Work out the finished part from the listing and answer in its coordinate system (mm). A direction names the side the tool comes from. Round coordinates to 2 decimals unless told otherwise and drop trailing zeros. Write each loop counter-clockwise with the first axis right and the second up, starting at its lowest first coordinate (ties: lowest second). Pieces come first, ordered by that corner, then holes. Notation, with made-up numbers: M 75.5,24.25 L 96.5,24.25 A26 ccw 96.5,39.25 Z; hole C 42.25,6 d4. An arc over 180 degrees is marked long. Answer in a Markdown table with one row per item.
```python
from build123d import *

# Parameters (mm, degrees)
BOSS_EXTRUDE1_DEPTH     = 15
SKETCH2_R               = 10
CUT_EXTRUDE1_DEPTH      = 109.972473589
SKETCH3_W               = 40
SKETCH3_H               = 10
BOSS_EXTRUDE2_DEPTH     = 55
CUT_EXTRUDE2_DEPTH      = 136.738719605
CUT_EXTRUDE2_DEPTH_BACK = 136.738719605


with BuildPart() as part:
    # Sketch1 → Boss-Extrude1 (new body)
    with BuildSketch(Plane(origin=(0, 0, 0), x_dir=(1, 0, 0), z_dir=(0, 1, 0))):
        with BuildLine():
            Line((0, 25), (80, 25))
            ThreePointArc((80, 25), (105, 0), (80, -25))
            Line((80, -25), (0, -25))
            ThreePointArc((0, -25), (-25, 0), (0, 25))
        make_face()
    extrude(amount=BOSS_EXTRUDE1_DEPTH)

    # Sketch2 → Cut-Extrude1 (cut, through all)
    with BuildSketch(Plane(origin=(0, 15, 0), x_dir=(1, 0, 0), z_dir=(0, 1, 0))):
        with Locations(Location((0, 0, 0), (0, 0, 270))):
            Circle(SKETCH2_R)
        with Locations(Location((80, 0, 0), (0, 0, 90))):
            Circle(SKETCH2_R)
    extrude(amount=-CUT_EXTRUDE1_DEPTH, mode=Mode.SUBTRACT)

    # Sketch3 → Boss-Extrude2 (add)
    with BuildSketch(Plane(origin=(0, 15, 0), x_dir=(1, 0, 0), z_dir=(0, 1, 0))):
        with Locations((40, 20)):
            Rectangle(SKETCH3_W, SKETCH3_H)
        with Locations((40, -20)):
            Rectangle(SKETCH3_W, SKETCH3_H)
    extrude(amount=BOSS_EXTRUDE2_DEPTH)

    # Sketch4 → Cut-Extrude2 (cut, two sides)
    with BuildSketch(Plane.XY.offset(25)) as cut_extrude2_sk:
        with BuildLine():
            ThreePointArc((30, 50), (40, 40), (50, 50))
            Line((50, 50), (30, 50))
        make_face()
        with BuildLine():
            Line((30, 50), (50, 50))
            ThreePointArc((50, 50), (40, 60), (30, 50))
        make_face()
        with BuildLine():
            ThreePointArc((40, 70), (54.142135624, 64.142135624), (60, 50))
            Line((60, 50), (60, 70))
            Line((60, 70), (40, 70))
        make_face()
        with BuildLine():
            ThreePointArc((20, 50), (25.857864376, 64.142135624), (40, 70))
            Line((40, 70), (20, 70))
            Line((20, 70), (20, 50))
        make_face()
    extrude(amount=CUT_EXTRUDE2_DEPTH, mode=Mode.SUBTRACT)
    extrude(cut_extrude2_sk.sketch, amount=-CUT_EXTRUDE2_DEPTH_BACK, mode=Mode.SUBTRACT)


solid = part.part
```
1. A tool of negligible diameter and unlimited length cuts with its end or side. For faces 1 (the flat face through (40, 36, -15)), 2 (the flat face through (39, 27, -25)), 3 (the flat face through (20, 32, -20)), 4 (the cylindrical face through (37.83, 40.24, 20.07)), 5 (the flat face through (60, 32, 20)), from which of +Z, -Z, +X, -X, +Y, -Y can it reach the whole face along a straight path? Write none if from no direction.
Calculated:
| item | result |
|---|---|
| face 1 | +X, -X, +Y |
| face 2 | -Z, +X, -X, +Y, -Y |
| face 3 | +Z, -Z, -X, +Y |
| face 4 | +Z, -Z |
| face 5 | +Z, -Z, +X, +Y |
2. The part is cut by section C-C (y = 9). Determine the outline of the cut face in (x, z).
Calculated:
| item | result |
|---|---|
| outline | M 0,-25 L 80,-25 A25 ccw 80,25 L 0,25 A25 ccw Z; hole C 0,0 d20; hole C 80,0 d20 |
3. Determine the mould class of faces 6 (the flat face through (40, 36, 15)), 7 (the cylindrical face through (70.085, 7.605, 1.302)), 8 (the flat face through (20, 32, 20)) for opening direction X: released by +X, released by -X, zero draft, split by the parting line, or undercut.
Calculated:
| item | result |
|---|---|
| face 6 | zero draft |
| face 7 | undercut |
| face 8 | released by -X |
4. Consider line 1 along X through (y, z) = (9.5, 0); line 2 along Y through (x, z) = (40, 22.75); line 3 along X through (y, z) = (13.5, -8.5). Determine where each line is inside the solid, lowest interval first. Write a range as from..to.
Calculated:
| item | result |
|---|---|
| line 1 | x = -25..-10, 10..70, 90..105 |
| line 2 | y = 0..40, 60..70 |
| line 3 | x = -23.51..-5.27, 5.27..74.73, 85.27..103.51 |
5. The part is cut by section D-D (x = 47.5). Determine the outline of the cut face in (y, z), plus the area to 3 significant figures.
Calculated:
| item | result |
|---|---|
| outline | M 0,-25 L 43.39,-25 L 43.39,-15 L 15,-15 L 15,15 L 43.39,15 L 43.39,25 L 0,25 Z; M 56.61,-25 L 68.54,-25 L 68.54,-15 L 56.61,-15 Z; M 56.61,15 L 68.54,15 L 68.54,25 L 56.61,25 Z |
| area | 1,560 mm² |
6. The part is cut by section B-B (x = 74). Determine the outline of the cut face in (y, z), plus the area to 3 significant figures.
Calculated:
| item | result |
|---|---|
| outline | M 0,-25 L 15,-25 L 15,-8 L 0,-8 Z; M 0,8 L 15,8 L 15,25 L 0,25 Z |
| area | 510 mm² |
7. Given pin 1 (12 mm diameter, centred on y = 32.5, z = 14, fed in from -X); pin 2 (5 mm diameter, centred on y = 41, z = -18, fed in from +X); pin 3 (25 mm diameter, centred on x = 41, z = -11, fed in from +Y); pin 4 (6 mm diameter, centred on x = -8.5, z = -3, fed in from +Y), each flat-ended and moving along its own axis, determine where each tip first touches the part or whether it passes through.
Calculated:
| item | result |
|---|---|
| pin 1 | stops at x = 20 |
| pin 2 | stops at x = 60 |
| pin 3 | stops at y = 70 |
| pin 4 | stops at y = 15 |
8. The part is cut by section A-A (z = 0). Determine the outline of the cut face in (x, y).
Calculated:
| item | result |
|---|---|
| outline | M -25,0 L -10,0 L -10,15 L -25,15 Z; M 10,0 L 70,0 L 70,15 L 10,15 Z; M 90,0 L 105,0 L 105,15 L 90,15 Z |
